Here's how the part is built. I have some questions about the finished solid (model axes, mm). Face numbers are marked on the shaded views. A direction names the side the tool comes from. Round coordinates to 2 decimals unless told otherwise and drop trailing zeros. Order: outer loops, then holes, each group sorted by start corner. A loop starts at its lowest first (then second) coordinate and runs counter-clockwise, first axis right, second up.
```python
from build123d import *

# Parameters (mm, degrees)
SKETCH_1_W          = 15
SKETCH_1_H          = 15
SKETCH_1_W_2        = 12
SKETCH_1_H_2        = 12
EXTRUDE_2_DEPTH     = 66
SKETCH_3_R          = 4
CUT_EXTRUDE_1_DEPTH = 10
SKETCH_4_R          = 4
CUT_EXTRUDE_2_DEPTH = 10
SKETCH_5_R          = 4
CUT_EXTRUDE_3_DEPTH = 10
SKETCH_6_R          = 1.5
CUT_EXTRUDE_4_DEPTH = 10
SKETCH_7_R          = 1.5
CUT_EXTRUDE_5_DEPTH = 10
SKETCH_8_R          = 1.5
CUT_EXTRUDE_6_DEPTH = 10
SKETCH_9_R          = 4
CUT_EXTRUDE_7_DEPTH = 10


with BuildPart() as part:
    # ｽｹｯﾁ1 → ﾎﾞｽ - 押し出し2 (new body)
    with BuildSketch(Plane.XY):
        with Locations((0.489915859, 0.232626086)):
            Rectangle(SKETCH_1_W, SKETCH_1_H)
        with Locations((0.489915859, 0.232626086)):
            Rectangle(SKETCH_1_W_2, SKETCH_1_H_2, mode=Mode.SUBTRACT)
    extrude(amount=EXTRUDE_2_DEPTH)

    # ｽｹｯﾁ3 → ｶｯﾄ - 押し出し1 (cut)
    with BuildSketch(Plane(origin=(0, 7.732626086, 0), x_dir=(1, 0, 0), z_dir=(0, 1, 0))):
        with Locations((0.489915859, -58.5)):
            Circle(SKETCH_3_R)
    extrude(amount=-CUT_EXTRUDE_1_DEPTH, mode=Mode.SUBTRACT)

    # ｽｹｯﾁ4 → ｶｯﾄ - 押し出し2 (cut)
    with BuildSketch(Plane(origin=(0, 7.732626086, 0), x_dir=(1, 0, 0), z_dir=(0, 1, 0))):
        with Locations((0.489915859, -7.5)):
            Circle(SKETCH_4_R)
    extrude(amount=-CUT_EXTRUDE_2_DEPTH, mode=Mode.SUBTRACT)

    # ｽｹｯﾁ5 → ｶｯﾄ - 押し出し3 (cut)
    with BuildSketch(Plane.ZY.offset(7.010084141)):
        with Locations((33, 0.232626086)):
            Circle(SKETCH_5_R)
    extrude(amount=-CUT_EXTRUDE_3_DEPTH, mode=Mode.SUBTRACT)

    # ｽｹｯﾁ6 → ｶｯﾄ - 押し出し4 (cut)
    with BuildSketch(Plane(origin=(7.989915859, 0, 0), x_dir=(0, 0, -1), z_dir=(1, 0, 0))):
        with Locations((-33, 0.232626086)):
            Circle(SKETCH_6_R)
    extrude(amount=-CUT_EXTRUDE_4_DEPTH, mode=Mode.SUBTRACT)

    # ｽｹｯﾁ7 → ｶｯﾄ - 押し出し5 (cut)
    with BuildSketch(Plane.XZ.offset(7.267373914)):
        with Locations((0.489915859, 58.5)):
            Circle(SKETCH_7_R)
        with Locations((0.489915859, 7.5)):
            Circle(SKETCH_7_R)
    extrude(amount=-CUT_EXTRUDE_5_DEPTH, mode=Mode.SUBTRACT)

    # ｽｹｯﾁ8 → ｶｯﾄ - 押し出し6 (cut)
    with BuildSketch(Plane.ZY.offset(7.010084141)):
        with Locations((45.6, 0.232626086)):
            Circle(SKETCH_8_R)
        with Locations((20.4, 0.232626086)):
            Circle(SKETCH_8_R)
    extrude(amount=-CUT_EXTRUDE_6_DEPTH, mode=Mode.SUBTRACT)

    # ｽｹｯﾁ9 → ｶｯﾄ - 押し出し7 (cut)
    with BuildSketch(Plane(origin=(7.989915859, 0, 0), x_dir=(0, 0, -1), z_dir=(1, 0, 0))):
        with Locations((-20.4, 0.232626086)):
            Circle(SKETCH_9_R)
        with Locations((-45.6, 0.232626086)):
            Circle(SKETCH_9_R)
    extrude(amount=-CUT_EXTRUDE_7_DEPTH, mode=Mode.SUBTRACT)


solid = part.part
```
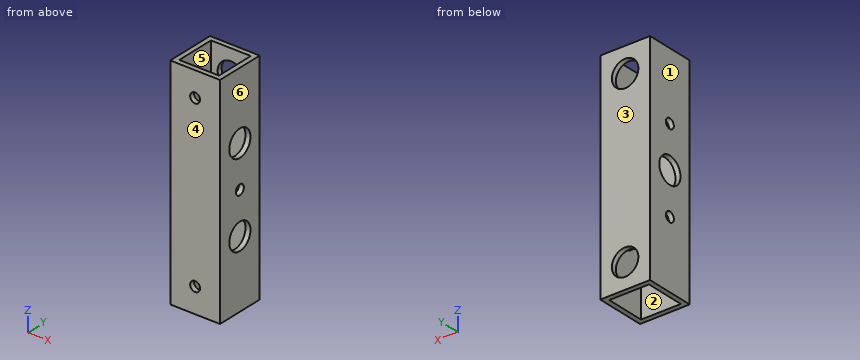
1. On a 3-axis mill with a long thin cutter (end or side, diameter ignored), from which of +Z, -Z, +X, -X, +Y, -Y can I reach the whole of each face in a straight line? I mean the marked faces 1 and 2. Say none if no direction works.
Evaluation:
face 1: +Z, -Z, -X, +Y, -Y
face 2: +Z, -Z
2. I'm going to push flat-ended pins straight in: P1, Ø5, axis at y = 0.23, z = 33, coming from the -X side; P2, Ø2.5, axis at y = 0.23, z = 20.4, coming from the +X side; P3, Ø6.5, axis at x = 0.49, z = 7.5, coming from the +Y side. Where does each tip first touch, or does it pass through?
Evaluation:
P1: stops at x = 6.49
P2: passes through
P3: stops at y = -5.77
3. If we section it at A-A, the plane z = 33: Write out the boundary of the cut face in (x, y).
Evaluation:
outline: (-7.01, -7.27) - (7.99, -7.27) - (7.99, -1.27) - (6.49, -1.27) - (6.49, -5.77) - (-5.51, -5.77) - (-5.51, -3.77) - (-7.01, -3.77) - close; (-7.01, 4.23) - (-5.51, 4.23) - (-5.51, 6.23) - (6.49, 6.23) - (6.49, 1.73) - (7.99, 1.73) - (7.99, 7.73) - (-7.01, 7.73) - close
4. If we mould it in two halves opening along Y, with no side actions, what happens to the marked faces 3, 4, 5 and 6? For each: released by +Y, released by -Y, zero draft, split by the parting line, or undercut.
Evaluation:
face 3: released by +Y
face 4: released by -Y
face 5: undercut
face 6: zero draft
5. If we section it at B-B, the plane y = 1: State how many separate pieces and enclosed holes the cut face has, and give its area (3 significant figures).
Evaluation:
separate pieces: 8
enclosed holes: 0
area: 151 mm2
6. I need wall thicknesses on probe 1 along X at (y, z) = (-3.75, 50); probe 2 along Y at (x, z) = (0, 29); probe 3 along Y at (x, z) = (-5.9, 33). Which ranges of each line are inside material? Lowest first, please.
Evaluation:
probe 1: x = -7.01 to -5.51, 6.49 to 7.99
probe 2: y = -7.27 to -5.77, 6.23 to 7.73
probe 3: y = -7.27 to -3.77, 4.23 to 7.73
